Can you work these out from the drawing? Everything is in mm from the part's minimum corner. A direction names the side the tool comes from. Coordinates: 2 decimals unless noted, no trailing zeros. Write each loop counter-clockwise with the first axis right and the second up, starting at its lowest first coordinate (ties: lowest second). Pieces come first, ordered by that corner, then holes. Notation, with made-up numbers: (-30.5, 31) -> (3.5, 31) arc R19 ccw to (3.5, 67) -> close; hole circle Ø10 at (52.25, -4.75). An arc over 180 degrees is marked (long way). Use a Markdown table: item, result. Add a question column.
Item 1: Imagine slicing it at C-C, the plane z = 49. Write out the boundary of the cut face in (x, y).
Item 2: If I drill on line 1 along Z through (x, y) = (6.25, 13.75); line 2 along Y through (x, z) = (3.5, 31); line 3 along Y through (x, z) = (8.75, 17), over which ranges is the centre line in solid material (lowest first)? Write a range as from..to.
Item 3: On a 3-axis mill with a long thin cutter (end or side, diameter ignored), from which of +Z, -Z, +X, -X, +Y, -Y can I reach the whole of each face in a straight line? I mean the marked faces 1 and 2. Say none if no direction works.
Item 4: Will these pins go through, and if not, where does the flat tip stop? pin 1 Ø5 at (x, z) = (12, 31.5) entering from -Y; pin 2 Ø4 at (y, z) = (11, 37) entering from -X; pin 3 Ø4 at (x, z) = (2, 9.5) entering from -Y.
Item 5: Imagine slicing it at A-A, the plane y = 7.6. Write out the boundary of the cut face in (x, z), and give its area (3 significant figures).
Item 6: Imagine slicing it at D-D, the plane z = 64. Write out the boundary of the cut face in (x, y), and give its area (3 significant figures).
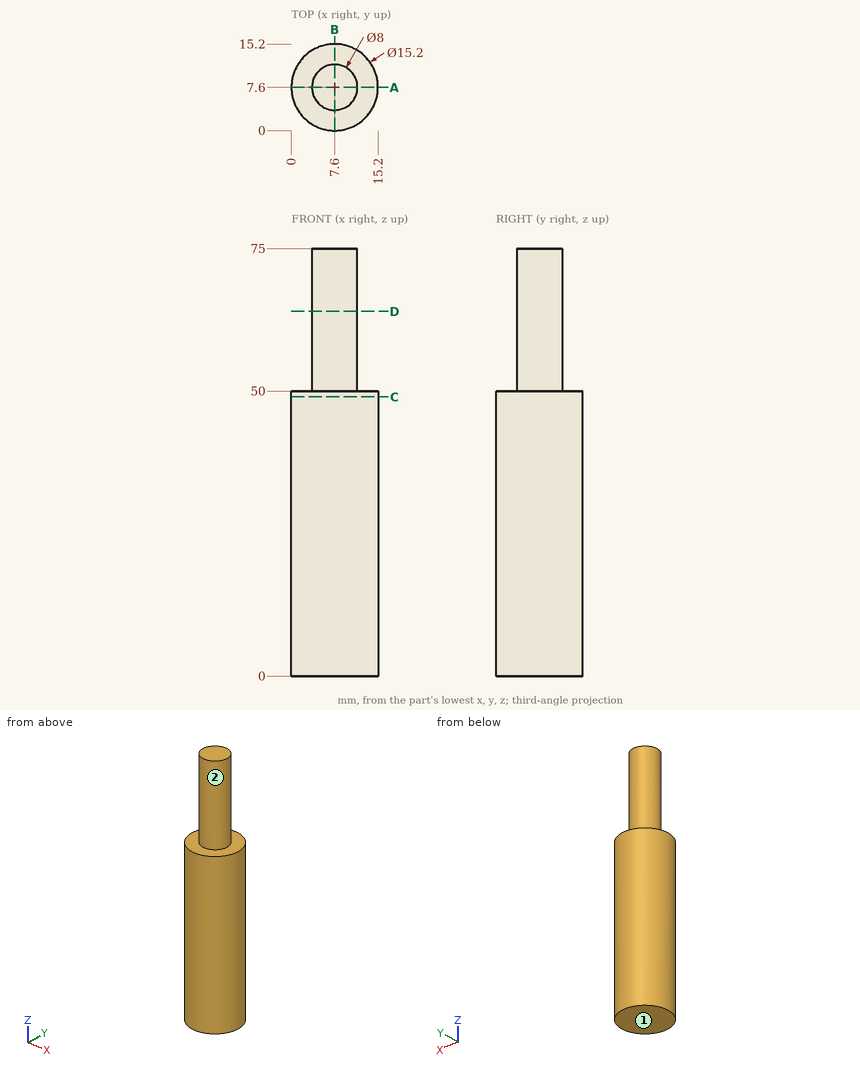
Ans:
| question | item | result |
|---|---|---|
| 1 | outline | circle Ø15.2 at (7.6, 7.6) |
| 2 | line 1 | z = 0..50 |
| 2 | line 2 | y = 1.2..14 |
| 2 | line 3 | y = 0.09..15.11 |
| 3 | face 1 | -Z, +X, -X, +Y, -Y |
| 3 | face 2 | +Z |
| 4 | pin 1 | stops at y = 0.24 |
| 4 | pin 2 | stops at x = 0.13 |
| 4 | pin 3 | stops at y = 0.91 |
| 5 | outline | (0, 0) -> (15.2, 0) -> (15.2, 50) -> (11.6, 50) -> (11.6, 75) -> (3.6, 75) -> (3.6, 50) -> (0, 50) -> close |
| 5 | area | 960 mm^2 |
| 6 | outline | circle Ø8 at (7.6, 7.6) |
| 6 | area | 50.3 mm^2 |
